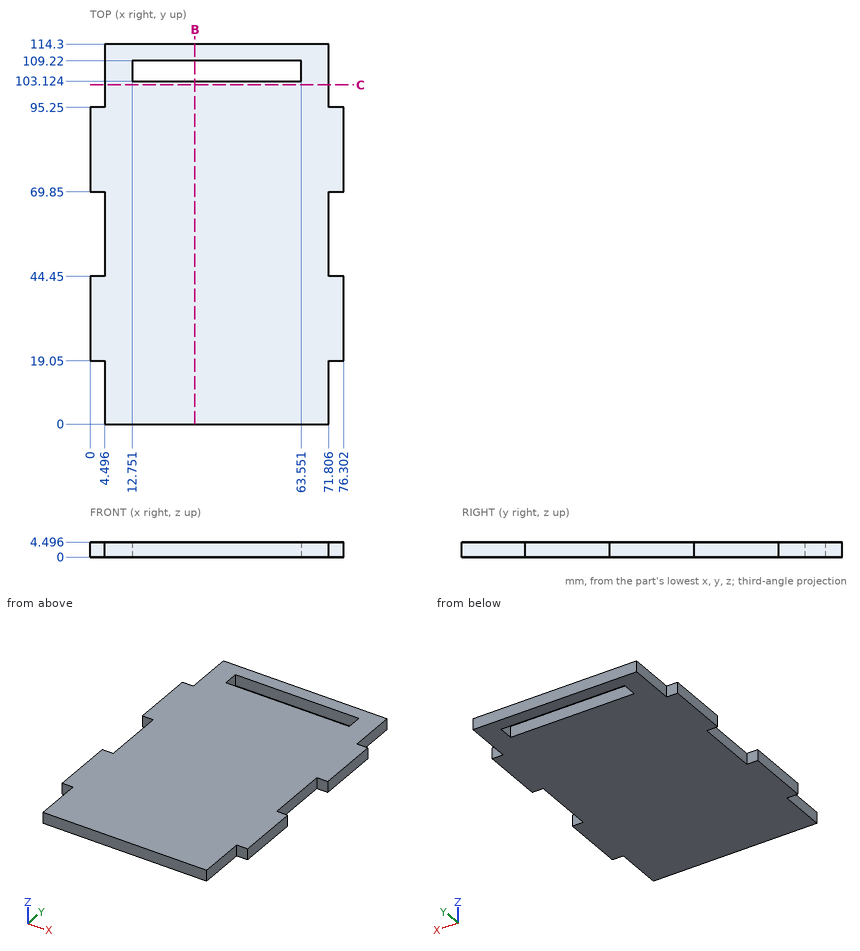
Input: dimensioned drawing with shaded views. Units: mm. Origin: part minimum x, y, z. Give positions to 0.01 mm unless a question says otherwise; leave off trailing zeros. Order: outer loops, then holes, each group sorted by start corner. A loop starts at its lowest first (then second) coordinate and runs counter-clockwise, first axis right, second up. Notation, with made-up numbers: (16.25, -23) -> (38.25, -23) arc R23 ccw to (38.25, -13) -> close; hole circle Ø1 at (-8, -17.5). An arc over 180 degrees is marked (long way). Use a Markdown table: item, result.
1) Section query B-B, the plane x = 31.5. Return the cut outline in (y, z) (1 decimal).
Answer list:
| item | result |
|---|---|
| outline | (0, 0) -> (103.1, 0) -> (103.1, 4.5) -> (0, 4.5) -> close; (109.2, 0) -> (114.3, 0) -> (114.3, 4.5) -> (109.2, 4.5) -> close |
2) Contact query for flat-ended pins moving along their axis: P1, Ø2, axis at y = 58, z = 1.5, coming from the -X side; P2, Ø1.3, axis at x = 2, z = 1.5, coming from the +Y side; P3, Ø2, axis at x = 2.5, z = 2, coming from the -Y side. Output: stop coordinate, or through.
Answer list:
| item | result |
|---|---|
| P1 | x = 4.5 |
| P2 | y = 95.25 |
| P3 | y = 19.05 |
3) Ray query, line 1 along Y through (x, z) = (26.5, 1.65); line 2 along X through (y, z) = (54, 3.05) (1 decimal); line 3 along Y through (x, z) = (73.5, 3.5). Return the intervals inside material, ascending. Write a range as [from, to].
Answer list:
| item | result |
|---|---|
| line 1 | [0, 103.12], [109.22, 114.3] |
| line 2 | [4.5, 71.8] |
| line 3 | [19.05, 44.45], [69.85, 95.25] |
4) Section query C-C, the plane y = 102. Return the cut outline in (x, z) (1 decimal).
Answer list:
| item | result |
|---|---|
| outline | (4.5, 0) -> (71.8, 0) -> (71.8, 4.5) -> (4.5, 4.5) -> close |
